```python
from build123d import *

# Parameters (mm, degrees)
F0_R           = 2
F1_DEPTH       = 75
F2_W           = 3
F2_H           = 25
F3_DEPTH       = 12.5
F5_D           = 6
F5_CSINK_D     = 8
F5_CSINK_ANGLE = 90


with BuildPart() as f1:
    # F0 (on Top) → F1 (new body)
    with BuildSketch(Plane.XY):
        with BuildLine():
            Line((30, 1.5), (2.5980762114, 1.5))
            ThreePointArc((2.5980762114, 1.5), (-3, 0), (2.5980762114, -1.5))
            Line((2.5980762114, -1.5), (30, -1.5))
            Line((30, -1.5), (30, 1.5))
        make_face()
        Circle(F0_R, mode=Mode.SUBTRACT)
    extrude(amount=F1_DEPTH)

    # F2 (on Front) → F3 (cut, symmetric)
    with BuildSketch(Plane.XZ):
        with Locations((-1.5, 12.5)):
            Rectangle(F2_W, F2_H)
        with Locations((1.5, 12.5)):
            Rectangle(F2_W, F2_H)
        with Locations((-1.5, 62.5)):
            Rectangle(F2_W, F2_H)
        with Locations((1.5, 62.5)):
            Rectangle(F2_W, F2_H)
    extrude(amount=F3_DEPTH, both=True, mode=Mode.SUBTRACT)

    # F5 (through all)
    with Locations(Plane(origin=(0, 1.5, 0), x_dir=(-1, 0, 0), z_dir=(0, 1, 0))):
        with Locations((-16.5, 65), (-24, 37.5), (-16.5, 10)):
            CounterSinkHole(F5_D / 2, F5_CSINK_D / 2, counter_sink_angle=F5_CSINK_ANGLE)


solid = f1.part
```
Input: part model. Units: mm. Frame: model coordinates. A direction names the side the tool comes from. Give positions to 0.01 mm unless a question says otherwise; leave off trailing zeros. Order: outer loops, then holes, each group sorted by start corner. A loop starts at its lowest first (then second) coordinate and runs counter-clockwise, first axis right, second up.
1. Section B-B on x = 16.5. Return the cut outline in (y, z), and give its area (3 significant figures).
Derived:
outline: (-1.5, 0) - (1.5, 0) - (1.5, 6) - (0.5, 7) - (-1.5, 7) - close; (-1.5, 13) - (0.5, 13) - (1.5, 14) - (1.5, 61) - (0.5, 62) - (-1.5, 62) - close; (-1.5, 68) - (0.5, 68) - (1.5, 69) - (1.5, 75) - (-1.5, 75) - close
area: 187 mm2
2. Mould query, pull axis Z, two halves, no side actions, for faces 6 (the flat face through (16, 0, 0)), 7 (the flat face through (16, 0, 75)), 8 (the flat face through (16, -1.5, 37)), 9 (the conical face through (13, 1, 65)). Classes: released by +Z, released by -Z, zero draft, split by the parting line, or undercut.
Derived:
face 6: released by -Z
face 7: released by +Z
face 8: zero draft
face 9: undercut
3. Section C-C on x = 24. Return the cut outline in (y, z), and give its area (3 significant figures).
Derived:
outline: (-1.5, 0) - (1.5, 0) - (1.5, 33.5) - (0.5, 34.5) - (-1.5, 34.5) - close; (-1.5, 40.5) - (0.5, 40.5) - (1.5, 41.5) - (1.5, 75) - (-1.5, 75) - close
area: 206 mm2
4. Section A-A on z = 37.5. Return the cut outline in (x, y), and give its area (3 significant figures).
Derived:
outline: (2.6, -1.5) - (21, -1.5) - (21, 0.5) - (20, 1.5) - (2.6, 1.5) arc R3 ccw (long way) to start; (27, -1.5) - (30, -1.5) - (30, 1.5) - (28, 1.5) - (27, 0.5) - close; hole circle Ø4 at (0, 0)
area: 78.1 mm2
5. Section D-D on z = 65. Return the cut outline in (x, y), and give its area (3 significant figures).
Derived:
outline: (3, -1.5) - (13.5, -1.5) - (13.5, 0.5) - (12.5, 1.5) - (3, 1.5) - close; (19.5, -1.5) - (30, -1.5) - (30, 1.5) - (20.5, 1.5) - (19.5, 0.5) - close
area: 62.0 mm2
6. Material intervals for L1, parallel to Z at x = 16.5, y = -0.75; L2, parallel to Z at x = 24, y = -0.3; L3, parallel to X at y = -1, z = 65, sorted ascending.
Derived:
L1: z = 0 to 7, 13 to 62, 68 to 75
L2: z = 0 to 34.5, 40.5 to 75
L3: x = 3 to 13.5, 19.5 to 30
7. Pin query (flat end, axial travel): pin 1 (2 mm diameter, centred on x = 0.5, z = 64.5, fed in from +Y); pin 2 (13.5 mm diameter, centred on x = 22, z = 46, fed in from -Y); pin 3 (1 mm diameter, centred on y = -2, z = 44, fed in from -X); pin 4 (8 mm diameter, centred on x = 17, z = 48.5, fed in from +Y). Return the tip coordinate at first contact, or that it passes through.
Derived:
pin 1: passes through
pin 2: stops at y = -1.5
pin 3: stops at x = -2.6
pin 4: stops at y = 1.5
8. Reachability of faces 1 (the flat face through (16, 1.5, 37)), 2 (the flat face through (3, 0, 12)), 3 (the cylindrical face through (15.85, -0.51, 62.07)), 4 (the cylindrical face through (0, -2, 37)), 5 (the flat face through (3, 0, 62)) from +Z, -Z, +X, -X, +Y, -Y: full face, straight path, thin tool, end or side. Return the list, or none.
Derived:
face 1: +Z, -Z, +X, +Y
face 2: -Z, -X, +Y, -Y
face 3: +Y, -Y
face 4: +Z, -Z
face 5: +Z, -X, +Y, -Y
